Part model, mm, in its own coordinate system. A direction names the side the tool comes from. Round coordinates to 2 decimals unless told otherwise and drop trailing zeros. Loops run counter-clockwise (first coordinate to the right, second up) from the corner with the lowest first, then second, coordinate; pieces in that order, holes last.
from build123d import *

# Parameters (mm, degrees)
F0_W     = 63.7512656803
F0_H     = 75
F0_W_2   = 76.2487343197
F1_DEPTH = 65
F2_R     = 15
F3_T     = 2.5


# Not quite as in the source:
# - a shell that OpenCascade refuses in one call is made with other operations: the cavity is built on its own and cut out


with BuildPart() as f1:
    # F0 (on Top) → F1 (new body)
    with BuildSketch(Plane.XY):
        with BuildLine():
            Line((-63.7512656803, -75), (-63.7512656803, 0))
            ThreePointArc((-63.7512656803, 0), (-101.2512656803, -37.5), (-63.7512656803, -75))
        make_face()
        with Locations((-31.8756328402, -37.5)):
            Rectangle(F0_W, F0_H)
        with Locations((38.1243671598, -37.5)):
            Rectangle(F0_W_2, F0_H)
        with BuildLine():
            ThreePointArc((76.2487343197, -75), (113.7487343197, -37.5), (76.2487343197, 0))
            Line((76.2487343197, 0), (76.2487343197, -75))
        make_face()
    extrude(amount=F1_DEPTH)

    # F2
    f2_edges = [f1.edges().sort_by_distance(p)[0] for p in [
        (-101.251266, -37.5, 65),
        (113.748734, -37.5, 0),
        (6.248734, -75, 65),
        (113.748734, -37.5, 65),
        (6.248734, 0, 65),
    ]]
    fillet(f2_edges, radius=F2_R)

    # F3: shell of thickness 2.5, made by hand


with BuildPart() as f3_core1:
    # F3_t2: copy of F1
    add(f1.part)

    # the walls: a layer under each face that stays
    f3_faces = [f3_core1.faces().sort_by_distance(p)[0] for p in [
        (-101.2512656803, -37.5, 32.5),
        (6.2487343197, 0, 32.5),
        (-96.8578673981, -37.5, 60.6066017178),
        (6.2487343197, -75, 32.5),
        (113.7487343197, -37.5, 32.5),
        (6.2487343197, -4.3933982822, 60.6066017178),
        (6.2487343197, -37.5, 65),
        (6.2487343197, -70.6066017178, 60.6066017178),
        (109.3553360375, -37.5, 60.6066017178),
    ]]
    thicken(f3_faces, amount=-F3_T, mode=Mode.SUBTRACT)


with BuildPart() as f1_1:
    add(f1.part)

    # what is left inside the walls is the cavity
    f3_cavity = [f3_core1.part.solids().sort_by_distance(p)[0] for p in [
        (6.248734, -45, 0.025),
    ]]
    add(f3_cavity, mode=Mode.SUBTRACT)


solid = f1_1.part
1) Slice it at C-C, the plane y = -37.5. Give the cut face in (x, z), then the cut area to 3 significant figures.
Values:
outline: (-101.25, 15) - (-98.75, 15) - (-98.75, 50) arc R12.5 cw to (-86.25, 62.5) - (98.75, 62.5) arc R12.5 cw to (111.25, 50) - (111.25, 15) - (113.75, 15) - (113.75, 50) arc R15 ccw to (98.75, 65) - (-86.25, 65) arc R15 ccw to (-101.25, 50) - close
area: 745 mm2
2) Mould opens along X. For faces 3 (the face through (113.74, -38.32, 32.25)), 4 (the face through (7.229, -68.935, 58.741)), 5 (the face through (5, -75, 32)) say: released by +X, released by -X, zero draft, split by the parting line, or undercut.
Values:
face 3: released by +X
face 4: undercut
face 5: zero draft
3) Wall check: line 1 along Y through (x, z) = (45, 23.5); line 2 along Z through (x, y) = (2.5, -22.5); line 3 along Y through (x, z) = (85, 30). Give the ranges that are in metal, low to high.
Values:
line 1: y = -75 to -72.5, -2.5 to 0
line 2: z = 62.5 to 65
line 3: y = -73.96 to -71.39, -3.61 to -1.04
4) Drop flat-ended pins along their axis: pin 1 Ø4 at (x, z) = (80, 30) entering from -Y; pin 2 Ø1 at (y, z) = (-11, 30) entering from +X; pin 3 Ø1 at (x, y) = (69, -60.5) entering from +Z; pin 4 Ø3 at (y, z) = (-40.5, 23) entering from +X. Give the stop position or say it passes through.
Values:
pin 1: stops at y = -74.96
pin 2: stops at x = 103.27
pin 3: stops at z = 65
pin 4: stops at x = 113.72
5) Tool access for faces 1 (the face through (5.27, -4.28, 60.49)), 2 (the face through (5.269, -6.065, 58.741)): list every direction of +Z, -Z, +X, -X, +Y, -Y with a clear straight run to the whole face (end or side of a thin tool).
Values:
face 1: +Z, +X, -X, +Y
face 2: -Z
6) Slice it at B-B, the plane z = 58. Give the cut face in (x, y), then the cut area to 3 significant figures.
Values:
outline: (-63.75, -72.69) - (76.25, -72.69) arc R35.19 ccw to (76.25, -2.31) - (-63.75, -2.31) arc R35.19 ccw to start; hole (-63.75, -69.6) - (76.25, -69.6) arc R32.1 ccw to (76.25, -5.4) - (-63.75, -5.4) arc R32.1 ccw to start
area: 1,520 mm2
7) Slice it at A-A, the plane x = 39. Give the cut face in (y, z), then the cut area to 3 significant figures.
Values:
outline: (-75, 15) - (-72.5, 15) - (-72.5, 50) arc R12.5 cw to (-60, 62.5) - (-15, 62.5) arc R12.5 cw to (-2.5, 50) - (-2.5, 15) - (0, 15) - (0, 50) arc R15 ccw to (-15, 65) - (-60, 65) arc R15 ccw to (-75, 50) - close
area: 395 mm2
